The listing builds one solid part. Answer for the finished solid, in the listing's coordinates (mm). Face numbers are marked on the shaded views. A direction names the side the tool comes from. Give positions to 0.01 mm unless a question says otherwise; leave off trailing zeros. Loops run counter-clockwise (first coordinate to the right, second up) from the corner with the lowest first, then second, coordinate; pieces in that order, holes last.
Item 1: Section D-D, the plane y = -8.5 is taken. Give the vertices of the cut face in (x, z).
Item 2: Section A-A, the plane x = 0 is taken. Give the vertices of the cut face in (y, z), and give its area (3 significant figures).
Item 3: A tool of negligible diameter and unlimited length cuts with its end or side. For the marked faces 5 and 6, from which of +Z, -Z, +X, -X, +Y, -Y can it reach the whole face along a straight path? Write none if from no direction.
Item 4: Section C-C, the plane z = 25 is taken. Give the vertices of the cut face in (x, y).
Item 5: The mould has two halves that part along X. Classify the marked faces 1, 2, 3 and 4: pulls with the +X half, pulls with the -X half, needs draft (parallel to the pull), parting line crosses it, or undercut.
Item 6: Consider line 1 along Z through (x, y) = (0, -49.5); line 2 along Z through (x, y) = (-5, -43.5); line 3 along Z through (x, y) = (0, -23.5). Determine where each line is inside the solid, lowest interval first.
Item 7: Each of these flat-tipped pins is pushed along its axis until it touches: pin 1 Ø18 at (y, z) = (-31, 4.5) entering from +X; pin 2 Ø2 at (y, z) = (-41, -8.5) entering from +X; pin 3 Ø4 at (x, z) = (-5.5, 0.5) entering from -Y. Where does it stop, or does it pass through?
Item 8: Section B-B, the plane y = -54 is taken. Give the vertices of the cut face in (x, z).
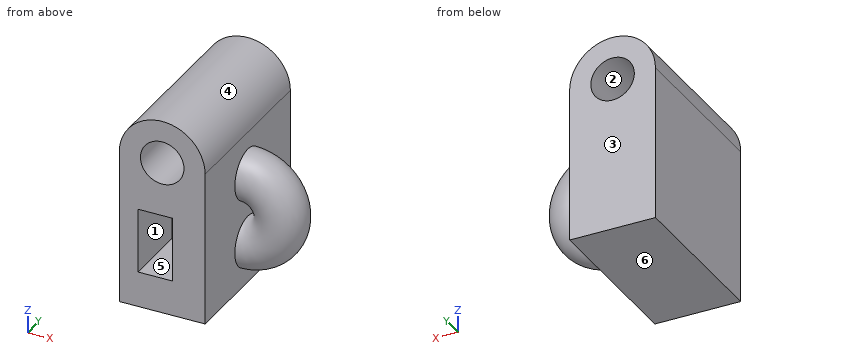
from build123d import *

# Parameters (mm, degrees)
F0_R     = 8.3642663508
F1_DEPTH = 63.5
F2_W     = 13.291940093
F2_H     = 24.8854812235
F3_DEPTH = 25.4
F4_R     = 9.7063550573
F5_ANGLE = 180


# Not quite as in the source:
# - a feature names something its author has since deleted; it is built from what else it names


with BuildPart() as f1:
    # F0 (on Front) → F1 (new body)
    with BuildSketch(Plane.XZ):
        with BuildLine():
            Line((-16.4914578199, -29.6862870455), (16.4914578199, -29.6862870455))
            Line((16.4914578199, -29.6862870455), (16.4914578199, 29.6862870455))
            ThreePointArc((16.4914578199, 29.6862870455), (0, 46.1777448654), (-16.4914578199, 29.6862870455))
            Line((-16.4914578199, 29.6862870455), (-16.4914578199, -29.6862870455))
        make_face()
        with Locations((0, 29.6862870455)):
            Circle(F0_R, mode=Mode.SUBTRACT)
    extrude(amount=F1_DEPTH)

    # F2 (on face) → F3 (cut)
    with BuildSketch(Plane.XZ.offset(63.5)):
        with Locations((-2.6479512453, -3.5954387859)):
            Rectangle(F2_W, F2_H)
    extrude(amount=-F3_DEPTH, mode=Mode.SUBTRACT)

    # F4 (on face) → F5 (revolve)
    with BuildSketch(Plane.YZ.offset(16.4914578199)):
        with Locations((-31.6691994667, 13.287819922)):
            Circle(F4_R)
    revolve(axis=Axis((16.4914578199, -31.75, 0), (0, 1, 0)), revolution_arc=F5_ANGLE)


solid = f1.part
Worked answers:
1. outline: (-16.49, -29.69) - (16.49, -29.69) - (16.49, 29.69) arc R16.49 ccw to (-16.49, 29.69) - close; hole circle Ø16.73 at (0, 29.69)
2. outline: (-63.5, -29.69) - (0, -29.69) - (0, 21.32) - (-63.5, 21.32) - (-63.5, 8.85) - (-38.1, 8.85) - (-38.1, -16.04) - (-63.5, -16.04) - close; (-63.5, 38.05) - (0, 38.05) - (0, 46.18) - (-63.5, 46.18) - close
2. area: 3,120 mm2
3. face 5: -Y
3. face 6: -Z, +X, -X, +Y, -Y
4. outline: (-16.49, -63.5) - (-6.93, -63.5) - (-6.93, 0) - (-16.49, 0) - close; (6.93, -63.5) - (16.49, -63.5) - (16.49, 0) - (6.93, 0) - close
5. face 1: undercut
5. face 2: undercut
5. face 3: needs draft
5. face 4: parting line crosses it
6. line 1: z = -29.69 to -16.04, 8.85 to 21.32, 38.05 to 46.18
6. line 2: z = -29.69 to -16.04, 8.85 to 22.98, 36.39 to 45.4
6. line 3: z = -29.69 to 21.32, 38.05 to 46.18
7. pin 1: stops at x = 39.49
7. pin 2: stops at x = 32.73
7. pin 3: stops at y = -38.1
8. outline: (-16.49, -29.69) - (16.49, -29.69) - (16.49, 29.69) arc R16.49 ccw to (-16.49, 29.69) - close; hole (-9.29, -16.04) - (4, -16.04) - (4, 8.85) - (-9.29, 8.85) - close; hole circle Ø16.73 at (0, 29.69)
